from build123d import *

# Parameters (mm, degrees)
SKETCH1_W           = 100.457
SKETCH1_H           = 39.4843
SKETCH1_R           = 1.59385
BOSS_EXTRUDE1_DEPTH = 1.6383
SKETCH3_R           = 3.1242
BOSS_EXTRUDE2_DEPTH = 10.668
SKETCH4_W           = 15.24
SKETCH4_H           = 5.08
BOSS_EXTRUDE3_DEPTH = 28.448


with BuildPart() as part:
    # Sketch1 → Boss-Extrude1 (new body)
    with BuildSketch(Plane(origin=(0, 0, 0), x_dir=(1, 0, 0), z_dir=(0, 1, 0))):
        with Locations((50.2285, 19.74215)):
            Rectangle(SKETCH1_W, SKETCH1_H)
        with Locations(Location((4.64185, 34.80435, 0), (0, 0, 90))):
            Circle(SKETCH1_R, mode=Mode.SUBTRACT)
        with Locations(Location((34.49955, 34.80435, 0), (0, 0, 90))):
            Circle(SKETCH1_R, mode=Mode.SUBTRACT)
        with Locations(Location((4.64185, 4.64185, 0), (0, 0, 90))):
            Circle(SKETCH1_R, mode=Mode.SUBTRACT)
        with Locations(Location((65.95745, 34.80435, 0), (0, 0, 90))):
            Circle(SKETCH1_R, mode=Mode.SUBTRACT)
        with Locations(Location((95.81515, 34.80435, 0), (0, 0, 90))):
            Circle(SKETCH1_R, mode=Mode.SUBTRACT)
        with Locations(Location((95.81515, 4.64185, 0), (0, 0, 90))):
            Circle(SKETCH1_R, mode=Mode.SUBTRACT)
    extrude(amount=BOSS_EXTRUDE1_DEPTH)

    # Sketch3 → Boss-Extrude2 (add)
    with BuildSketch(Plane(origin=(0, 1.6383, 0), x_dir=(1, 0, 0), z_dir=(0, 1, 0))):
        with Locations(Location((11.3792, 19.6215, 0), (0, 0, 90))):
            Circle(SKETCH3_R)
    extrude(amount=BOSS_EXTRUDE2_DEPTH)

    # Sketch4 → Boss-Extrude3 (add)
    with BuildSketch(Plane.XZ):
        with Locations((50.36185, -2.54)):
            Rectangle(SKETCH4_W, SKETCH4_H)
    extrude(amount=BOSS_EXTRUDE3_DEPTH)


solid = part.part
Model file for the job. Use its own axes, mm. A direction names the side the tool comes from. Give positions to 0.01 mm unless a question says otherwise; leave off trailing zeros. Loops run counter-clockwise (first coordinate to the right, second up) from the corner with the lowest first, then second, coordinate; pieces in that order, holes last.
1) Flat gauge pins, fed straight in: pin 1 Ø8 at (x, y) = (41.5, 2.5) entering from -Z; pin 2 Ø4 at (y, z) = (-3.5, -35.5) entering from +X; pin 3 Ø2.5 at (y, z) = (-13.5, -3.5) entering from -X; pin 4 Ø12 at (x, z) = (35.5, -18) entering from -Y. Where does each tip first touch, or does it go through?
2) Wall check: line 1 (Y direction, x = 45.5, z = -30); line 2 (X direction, y = -5.5, z = -2); line 3 (X direction, y = 2, z = -19.5). Give the ranges that are in metal, low to high.
3) Tool access for faces 5 (the cylindrical face through (13.28, 6.9, -17.14)), 6 (the cylindrical face through (4.572, 0.808, -33.212)), 7 (the flat face through (50, -10, 0)), 8 (the flat face through (50, -14, -5.08)), 9 (the flat face through (42.742, -14, -3)): list every direction of +Z, -Z, +X, -X, +Y, -Y with a clear straight run to the whole face (end or side of a thin tool).
4) Saw through at D-D (y = 7). Write the cut outline in (x, z), plus the area to 3 significant figures.
5) Saw through at B-B (y = -23.5). Write the cut outline in (x, z), plus the area to 3 significant figures.
6) Pull direction X, two halves, no side cores. Call faces 1 (the cylindrical face through (94.235, 0.808, -34.597)), 2 (the cylindrical face through (4.16, 0.81, -6.16)), 3 (the flat face through (50, 0, -20)), 4 (the flat face through (57.982, -14, -3)): +X half, -X half, draft (parallel to the pull), parting line (faces both ways), or undercut.
7) Saw through at C-C (z = -30.5). Write the cut outline in (x, y).
8) Saw through at A-A (x = 9.5). Write the cut outline in (y, z), plus the area to 3 significant figures.
Answer block:
1. pin 1: stops at z = -39.48
1. pin 2: passes through
1. pin 3: stops at x = 42.74
1. pin 4: stops at y = 0
2. line 1: y = 0 to 1.64
2. line 2: x = 42.74 to 57.98
2. line 3: x = 8.26 to 14.5
3. face 5: +Y
3. face 6: +Y, -Y
3. face 7: +Z, +X, -X, +Y, -Y
3. face 8: -Z, +X, -X, -Y
3. face 9: +Z, -Z, -X, -Y
4. outline: circle Ø6.25 at (11.38, -19.62)
4. area: 30.7 mm2
5. outline: (42.74, -5.08) - (57.98, -5.08) - (57.98, 0) - (42.74, 0) - close
5. area: 77.4 mm2
6. face 1: undercut
6. face 2: undercut
6. face 3: draft
6. face 4: +X half
7. outline: (0, 0) - (100.46, 0) - (100.46, 1.64) - (0, 1.64) - close
8. outline: (0, -39.48) - (1.64, -39.48) - (1.64, -22.12) - (12.31, -22.12) - (12.31, -17.13) - (1.64, -17.13) - (1.64, 0) - (0, 0) - close
8. area: 118 mm2
